The model under review builds one solid part; all positions refer to its coordinate system, in mm. A direction names the side the tool comes from. Round coordinates to 2 decimals unless told otherwise and drop trailing zeros. Loops run counter-clockwise (first coordinate to the right, second up) from the corner with the lowest first, then second, coordinate; pieces in that order, holes last. Notation, with made-up numbers: M 34,44 L 55,44 A26 cw 55,74 Z; hole C 16.25,36 d9. An arc over 180 degrees is marked long. Answer as a JSON object with one key per item and string values. Group by question number.
Item 1: Insertion check: P1, Ø16.5, axis at y = 2, z = -2, coming from the -X side; P2, Ø10, axis at y = -11, z = 5.5, coming from the +X side; P3, Ø2, axis at y = 0, z = -9, coming from the -X side; P4, Ø8, axis at x = 7, z = -5.5, coming from the +Y side. Each pin has a flat end and moves straight along its axis. Give the tip position at first contact, or say it passes through.
Item 2: Consider section A-A (x = 4.5). Give the boundary of the cut face in (y, z).
Item 3: The part is to be moulded in two halves that separate along Y. For faces 1 (the face through (8.15, 0.05, 10.25)), 2 (the face through (-1.63, -9.4, 5.2)), 3 (the face through (3.186, -12.553, -6.529)), say which applies: +Y half, -Y half, draft (parallel to the pull), parting line (faces both ways), or undercut.
Item 4: Tool access review of faces 4 (the face through (8.155, 7.603, 6.527)), 5 (the face through (1.821, 9.711, 3.993)): name each direction out of +Z, -Z, +X, -X, +Y, -Y from which nothing blocks a thin tool from reaching the whole face with its end or side.
Item 5: To check wall thickness, follow line 1 (Y direction, x = 10.25, z = -7.25); line 2 (X direction, y = -1.75, z = 7.5); line 3 (X direction, y = -0.75, z = 0.75). State the ranges of each line that lie inside material, in increasing order.
Item 6: Consider section B-B (y = 0). State how many separate pieces and enclosed holes the cut face has, and give its area (3 significant figures).
```python
from build123d import *

# Parameters (mm, degrees)
FILLET1_R          = 2
SKETCH2_R          = 1.25
CUT_EXTRUDE1_DEPTH = 12.25
SKETCH3_R          = 2.5
CUT_EXTRUDE2_DEPTH = 7.25


with BuildPart() as part:
    # Sketch1 → Revolve1 (revolve)
    with BuildSketch(Plane(origin=(0, 0, 0), x_dir=(1, 0, 0), z_dir=(0, 1, 0))):
        Polygon((-1.630434783, 14.15), (7.869565217, 14.15), (10.619565217, 11.140476118), (10.619565217, 4), (14.619565217, 4), (14.619565217, 0), (13.372742768, 0), (5.369565217, 0), (5.369565217, 10.5), (-1.630434783, 10.5), align=None)
    revolve(axis=Axis((-12.391304348, 0, 0), (1, 0, 0)))

    # Fillet1
    fillet1_edges = [part.edges().sort_by_distance(p)[0] for p in [
        (14.619565217, 0, 4),
    ]]
    fillet(fillet1_edges, radius=FILLET1_R)

    # Sketch2 → Cut-Extrude1 (cut)
    with BuildSketch(Plane(origin=(10.619565217, 0, 0), x_dir=(0, 0, -1), z_dir=(1, 0, 0))):
        with Locations((0, 9)):
            Circle(SKETCH2_R)
        with Locations((6.363961031, 6.363961031)):
            Circle(SKETCH2_R)
        with Locations((9, 0)):
            Circle(SKETCH2_R)
        with Locations((6.363961031, -6.363961031)):
            Circle(SKETCH2_R)
        with Locations((0, -9)):
            Circle(SKETCH2_R)
        with Locations((-6.363961031, -6.363961031)):
            Circle(SKETCH2_R)
        with Locations((-9, 0)):
            Circle(SKETCH2_R)
        with Locations((-6.363961031, 6.363961031)):
            Circle(SKETCH2_R)
    extrude(amount=-CUT_EXTRUDE1_DEPTH, mode=Mode.SUBTRACT)

    # Sketch3 → Cut-Extrude2 (cut)
    with BuildSketch(Plane.ZY.offset(1.630434783)):
        with Locations((0, 9)):
            Circle(SKETCH3_R)
        with Locations((6.363961031, 6.363961031)):
            Circle(SKETCH3_R)
        with Locations((9, 0)):
            Circle(SKETCH3_R)
        with Locations((6.363961031, -6.363961031)):
            Circle(SKETCH3_R)
        with Locations((0, -9)):
            Circle(SKETCH3_R)
        with Locations((-6.363961031, -6.363961031)):
            Circle(SKETCH3_R)
        with Locations((-9, 0)):
            Circle(SKETCH3_R)
        with Locations((-6.363961031, 6.363961031)):
            Circle(SKETCH3_R)
    extrude(amount=-CUT_EXTRUDE2_DEPTH, mode=Mode.SUBTRACT)


solid = part.part
```
Geometry results:
{
 "1": {"P1": "stops at x = -1.63", "P2": "stops at x = 10.62", "P3": "passes through", "P4": "stops at y = 14.07"},
 "2": {"outline": "C 0,0 d28.3; hole M -10.28,-2.15 A10.5 ccw -8.79,-5.75 A2.5 ccw -5.75,-8.79 A10.5 ccw -2.15,-10.28 A2.5 ccw 2.15,-10.28 A10.5 ccw 5.75,-8.79 A2.5 ccw 8.79,-5.75 A10.5 ccw 10.28,-2.15 A2.5 ccw 10.28,2.15 A10.5 ccw 8.79,5.75 A2.5 ccw 5.75,8.79 A10.5 ccw 2.15,10.28 A2.5 ccw -2.15,10.28 A10.5 ccw -5.75,8.79 A2.5 ccw -8.79,5.75 A10.5 ccw -10.28,2.15 A2.5 ccw Z"},
 "3": {"face 1": "undercut", "face 2": "draft", "face 3": "parting line"},
 "4": {"face 4": "+X, -X", "face 5": "-X"},
 "5": {"line 1": "y = -8.98 to -7.25, -5.48 to 5.48, 7.25 to 8.98", "line 2": "x = 5.62 to 10.62", "line 3": "x = 5.37 to 14.62"},
 "6": {"separate pieces": "3", "enclosed holes": "0", "area": "180 mm^2"}
}
